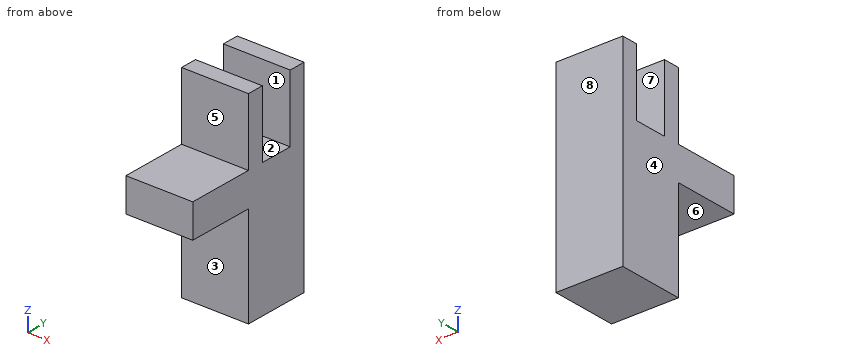
Autodesk Inventor part; units mm, degrees
ref_plane "YZ Plane" through (0, 0, 0) normal (1, 0, 0) x (0, 1, 0)
ref_plane "XZ Plane" through (0, 0, 0) normal (0, 1, 0) x (-1, 0, 0)
ref_plane "XY Plane" through (0, 0, 0) normal (0, 0, 1) x (1, 0, 0)
sketch "Sketch1" plane through (0, 0, 0) normal (1, 0, 0) x (0, 1, 0)
  line L0 (0, 0) -> (6.35, 0)
  line L1 (6.35, 0) -> (6.35, -6.35)
  line L2 (6.35, -6.35) -> (0, -6.35)
  line L3 (0, -6.35) -> (0, 0)
  dimension "d0" = 6.35
  dimension "d1" = 6.35
extrude "Extrusion1" add sketch "Sketch1" along normal blind 6.35
sketch "Sketch2" plane through (0, 0, 0) normal (0, 0, 1) x (1, 0, 0)
  line L0 (0, 0) -> (0, 6.35)
  line L1 (6.35, 6.35) -> (6.35, 0)
  line L2 (0, 4.7625) -> (6.35, 4.7625)
  line L3 (6.35, 4.7625) -> (6.35, 1.5875)
  line L4 (6.35, 1.5875) -> (0, 1.5875)
  line L5 (0, 1.5875) -> (0, 4.7625)
  line L6 (0, 0) -> (6.35, 0)
  line L7 (0, 1.5875) -> (0, 0)
  line L8 (0, 0) -> (6.35, 0)
  line L9 (6.35, 0) -> (6.35, 1.5875)
  line L10 (6.35, 4.7625) -> (6.35, 6.35)
  line L11 (0, 6.35) -> (6.35, 6.35)
  line L12 (0, 6.35) -> (0, 4.7625)
  line L13 (0, 6.35) -> (6.35, 6.35)
  dimension "d4" = 1.5875
  dimension "d5" = 3.175
extrude "Extrusion2" add sketch "Sketch2" along normal blind 6.35 contours L0 L4 L1 L6 | L0 L11 L1 L2
sketch "Sketch3" plane through (0, 0, -6.35) normal (0, -1, 0) x (1, 0, 0)
  line L0 (6.35, 0) -> (6.35, 12.7)
  line L1 (6.35, 6.35) -> (0, 6.35)
  line L2 (0, 6.35) -> (0, 3.175)
  line L3 (0, 3.175) -> (6.35, 3.175)
  line L4 (6.35, 3.175) -> (6.35, 6.35)
  dimension "d8" = 3.175
  dimension "d9" = 6.35
extrude "Extrusion3" add sketch "Sketch3" along normal blind 6.35
sketch "Sketch4" plane through (0, 0, -6.35) normal (0, 0, -1) x (-1, 0, 0)
  line L0 (0, 1.5875) -> (0, 0)
  line L1 (-6.35, 4.7625) -> (-6.35, 6.35)
  line L2 (0, 0) -> (-6.35, 0)
  line L3 (-6.35, 0) -> (-6.35, 6.35)
  line L4 (-6.35, 6.35) -> (0, 6.35)
  line L5 (0, 6.35) -> (0, 0)
extrude "Extrusion4" add sketch "Sketch4" along normal blind 6.35
properties part number "MonsterSupportHolder4"
Build history of the part. All positions in model axes, mm. Face numbers are marked on the shaded views. A direction names the side the tool comes from. Give positions to 0.01 mm unless a question says otherwise; leave off trailing zeros. Order: outer loops, then holes, each group sorted by start corner. A loop starts at its lowest first (then second) coordinate and runs counter-clockwise, first axis right, second up. Notation, with made-up numbers: M 18,-11.5 L 22,-11.5 A31 cw 22,16.5 Z; hole C -26.75,28 d5. An arc over 180 degrees is marked long. Put each result on its own line as item: value.
Item 1: Slice it at A-A, the plane z = 3. Write the cut outline in (x, y), plus the area to 3 significant figures.
From the geometry:
outline: M 0,0 L 6.35,0 L 6.35,1.59 L 0,1.59 Z; M 0,4.76 L 6.35,4.76 L 6.35,6.35 L 0,6.35 Z
area: 20.2 mm2
Item 2: Slice it at D-D, the plane z = -9.5. Write the cut outline in (x, y), plus the area to 3 significant figures.
From the geometry:
outline: M 0,0 L 6.35,0 L 6.35,6.35 L 0,6.35 Z
area: 40.3 mm2
Item 3: Flat gauge pin, fed straight in: pin 1 Ø1.5 at (x, z) = (3, -8) entering from -Y. Where does the tip first touch, or does it go through?
From the geometry:
pin 1: stops at y = 0
Item 4: Two-plate mould, pull along Y, no slides. Class the marked faces 1, 2, 3 and 4: +Y half, -Y half, draft (parallel to the pull), parting line (faces both ways), or undercut.
From the geometry:
face 1: undercut
face 2: undercut
face 3: -Y half
face 4: draft
Item 5: Slice it at C-C, the plane y = -1. Write the cut outline in (x, z) (3 decimals).
From the geometry:
outline: M 0,-3.175 L 6.35,-3.175 L 6.35,0 L 0,0 Z
Item 6: 3-axis set-ups, long thin cutter, end or side, ignore diameter. For the marked faces 5, 6, 7 and 8: which of +Z, -Z, +X, -X, +Y, -Y reach the whole face in a straight line?
From the geometry:
face 5: +Z, +X, -X, -Y
face 6: -Z, +X, -X, -Y
face 7: +Z, +X, -X
face 8: +Z, -Z, +X, -X, +Y
Item 7: Probe line 1 (Y direction, x = 1.5, z = 5); line 2 (Z direction, x = 5.5, y = -5.5) (3 decimals); line 3 (Z direction, x = 3.25, y = 1.75). List the from-to ranges inside material, lowest first. Write a range as [from, to].
From the geometry:
line 1: y = [0, 1.59], [4.76, 6.35]
line 2: z = [-3.175, 0]
line 3: z = [-12.7, 0]
